Source: CAD feature listing. Evaluate the final solid. Frame: model axes, mm. A direction names the side the tool comes from. Round coordinates to 2 decimals unless told otherwise and drop trailing zeros. Return JSON: item names as keys, results as strings. Group by question number.
```python
from build123d import *

# Parameters (mm, degrees)
SHELL1_T           = -1
SKETCH3_R          = 4
CUT_EXTRUDE3_DEPTH = 2
CIRPATTERN1_COUNT  = 30


with BuildPart() as part:
    # Sketch1 → Revolve1 (revolve)
    with BuildSketch(Plane.YZ, mode=Mode.PRIVATE) as revolve1_sk:
        with BuildLine():
            Line((0, 0), (13.02, 0))
            Line((13.02, 0), (13.02, 48.76))
            ThreePointArc((13.02, 48.76), (12.350127019, 51.26), (10.52, 53.090127019))
            Line((10.52, 53.090127019), (8.96, 53.990793439))
            Line((8.96, 53.990793439), (8.96, 57.190793439))
            Line((8.96, 57.190793439), (0, 57.190793439))
            Line((0, 57.190793439), (0, 0))
        make_face()
    revolve(revolve1_sk.sketch.rotate(Axis((0, -88.855588477, 0), (0, 1, 0)), 180), axis=Axis((0, -88.855588477, 0), (0, 1, 0)))

    # Shell1
    shell1_openings = [part.faces().sort_by_distance(p)[0] for p in [
        (0, 0, 0),
    ]]
    offset(amount=SHELL1_T, openings=shell1_openings, kind=Kind.INTERSECTION)

    # Sketch2 → Revolve2 (revolve)
    with BuildSketch(Plane.YZ, mode=Mode.PRIVATE) as revolve2_sk:
        Polygon((4.96, 53.41344317), (7.96, 53.41344317), (7.96, 55.41344317), (4.131572875, 55.41344317), (0.96, 52.241870294), (0.96, 30.585016045), (5.191572875, 26.35344317), (12.02, 26.35344317), (12.02, 28.35344317), (6.02, 28.35344317), (2.96, 31.41344317), (2.96, 51.41344317), align=None)
    revolve(revolve2_sk.sketch.rotate(Axis((0, -18.870621066, 0), (0, 1, 0)), 180), axis=Axis((0, -18.870621066, 0), (0, 1, 0)))

    # Sketch3 → Cut-Extrude3 (cut)
    with BuildSketch(Plane(origin=(0, 0.96, 0), x_dir=(-1, 0, 0), z_dir=(0, 1, 0))):
        with Locations(Location((41.38, 0, 0), (0, 0, 90))):
            Circle(SKETCH3_R)
    cut_extrude3 = extrude(amount=CUT_EXTRUDE3_DEPTH, mode=Mode.SUBTRACT)

    # CirPattern1: Cut-Extrude3 ×30 about axis
    cirpattern1_axis = Axis((0, 0, 0), (0, 1, 0))
    for i in range(1, CIRPATTERN1_COUNT):
        add(cut_extrude3.rotate(cirpattern1_axis, i * 360 / CIRPATTERN1_COUNT), mode=Mode.SUBTRACT)


solid = part.part
```
(1) Ray query, line 1 (Y direction, x = -20.5, z = 43); line 2 (X direction, y = 7.25, z = -32); line 3 (Z direction, x = -47.5, y = 5.75). Return the intervals inside material, ascending.
(2) Mould query, pull axis X, two halves, no side actions, for faces 1 (the face through (-34.2, 8.96, 42.1)), 2 (the face through (-54.942, 6.019, 7.214)). Classes: released by +X, released by -X, zero draft, split by the parting line, or undercut.
(3) Pin query (flat end, axial travel): pin 1 (13 mm diameter, centred on x = 27.69, z = -30.75, fed in from -Y); pin 2 (3 mm diameter, centred on y = 6.5, z = 9.5, fed in from +X); pin 3 (7 mm diameter, centred on x = 12.79, z = 39.35, fed in from -Y). Return the tip coordinate at first contact, or that it passes through.
(4) Set-up query: faces 3 (the face through (21, 12.02, 21)), 4 (the face through (-35.6, 1.95, -13.49)). Return all of +Z, -Z, +X, -X, +Y, -Y with unobstructed straight access to the full face (end or side cutting, diameter ignored); none if empty.
Answers follow:
{
 "1": {"line 1": "0.96 to 2.96, 12.02 to 13.02", "line 2": "-47.4 to -46.19, -45.24 to -42.77, 42.77 to 45.24, 46.19 to 47.4", "line 3": "-31.85 to -30.02, -28.54 to -24.43, 24.43 to 28.54, 30.02 to 31.85"},
 "2": {"face 1": "zero draft", "face 2": "undercut"},
 "3": {"pin 1": "y = 0.96", "pin 2": "x = 56.63", "pin 3": "y = 12.02"},
 "4": {"face 3": "none", "face 4": "-Y"}
}
